```python
from build123d import *

# Parameters (mm, degrees)
F2_R     = 1.55
F2_W     = 2
F2_H     = 2
F3_DEPTH = 1.5
F4_W     = 9
F4_H     = 5
F5_DEPTH = 3
F6_W     = 6
F6_H     = 6.7
F7_DEPTH = 2.5
F6_W_2   = 3.4
F6_H_2   = 3.4
F6_W_3   = 4.4
F6_H_3   = 4.4
F8_DEPTH = 1.5
F6_W_4   = 1.536496
F6_H_4   = 2.176703
F6_H_5   = 2.176704
F6_W_5   = 2.874283
F6_H_6   = 1.806834
F6_W_6   = 2.176703
F6_H_7   = 1.536496
F6_W_7   = 3.137013
F6_H_8   = 2.112682
F9_DEPTH = 2


with BuildPart() as f3:
    # F2 (on Top) → F3 (new body)
    with BuildSketch(Plane.XY):
        Polygon((18, 18), (-18, 18), (-18, 14.369573), (-18, 12.369573), (-18, 10.869573), (-18, 8.869573), (-18, 7.369573), (-18, 5.369573), (-18, 3.005002), (-18, 1.005002), (-18, -0.673528), (-18, -2.673528), (-18, -5.493983), (-18, -7.493983), (-18, -8.993983), (-18, -10.993983), (-18, -12.493983), (-18, -14.493983), (-18, -18), (18, -18), (18, -14.322089), (18, -12.322089), (18, -10.322089), (18, -8.322089), (18, -6.322089), (18, -4.322089), (18, 4.09024), (18, 6.09024), (18, 7.69024), (18, 9.69024), (18, 11.29024), (18, 13.29024), align=None)
        with Locations((-15.25, -15.25)):
            Circle(F2_R, mode=Mode.SUBTRACT)
        with Locations((15.25, -15.25)):
            Circle(F2_R, mode=Mode.SUBTRACT)
        with Locations((-15.25, 15.25)):
            Circle(F2_R, mode=Mode.SUBTRACT)
        with Locations((15.25, 15.25)):
            Circle(F2_R, mode=Mode.SUBTRACT)
        with Locations((-19, 13.369573)):
            Rectangle(F2_W, F2_H)
        with Locations((19, 12.29024)):
            Rectangle(F2_W, F2_H)
        with Locations((-19, 9.869573)):
            Rectangle(F2_W, F2_H)
        with Locations((19, 8.69024)):
            Rectangle(F2_W, F2_H)
        with Locations((-19, 6.369573)):
            Rectangle(F2_W, F2_H)
        with Locations((19, 5.09024)):
            Rectangle(F2_W, F2_H)
        with Locations((-19, 2.005002)):
            Rectangle(F2_W, F2_H)
        with Locations((19, -5.322089)):
            Rectangle(F2_W, F2_H)
        with Locations((-19, -1.673528)):
            Rectangle(F2_W, F2_H)
        with Locations((19, -9.322089)):
            Rectangle(F2_W, F2_H)
        with Locations((-19, -6.493983)):
            Rectangle(F2_W, F2_H)
        with Locations((19, -13.322089)):
            Rectangle(F2_W, F2_H)
        with Locations((-19, -9.993983)):
            Rectangle(F2_W, F2_H)
        with Locations((-19, -13.493983)):
            Rectangle(F2_W, F2_H)
    extrude(amount=F3_DEPTH)

    # F4 (on face) → F5 (join)
    with BuildSketch(Plane.XY.offset(1.5)):
        with Locations((-0.321198, 15.5)):
            Rectangle(F4_W, F4_H)
    extrude(amount=F5_DEPTH)

    # F6 (on face) → F7 (join)
    with BuildSketch(Plane(origin=(0, 0, 0), x_dir=(1, 0, 0), z_dir=(0, 0, -1))):
        with Locations((2.004663, -14.65)):
            Rectangle(F6_W, F6_H)
        with Locations((-7.845552, 14.65)):
            Rectangle(F6_W, F6_H)
        with Locations((7.711476, 14.65)):
            Rectangle(F6_W, F6_H)
    extrude(amount=F7_DEPTH)

    # F6 (on face) → F8 (join)
    with BuildSketch(Plane(origin=(0, 0, 0), x_dir=(1, 0, 0), z_dir=(0, 0, -1))):
        with Locations((-12.063461, -10.042248)):
            Rectangle(F6_W_2, F6_H_2)
        with Locations((-5.725725, -5.885644)):
            Rectangle(F6_W_3, F6_H_3)
        with Locations((6.013899, -6.527154)):
            Rectangle(F6_W_3, F6_H_3)
        with Locations((11.864845, -3.498852)):
            Rectangle(F6_W_2, F6_H_2)
        with Locations((12.121448, 7.278509)):
            Rectangle(F6_W_2, F6_H_2)
        with Locations((6.078051, 4.699263)):
            Rectangle(F6_W_3, F6_H_3)
        with Locations((-5.725725, 5.687943)):
            Rectangle(F6_W_3, F6_H_3)
        with Locations((-11.871008, 4.389598)):
            Rectangle(F6_W_2, F6_H_2)
    extrude(amount=F8_DEPTH)

    # F6 (on face) → F9 (join)
    with BuildSketch(Plane(origin=(0, 0, 0), x_dir=(1, 0, 0), z_dir=(0, 0, -1))):
        with Locations((-9.702151, -4.16677)):
            Rectangle(F6_W_4, F6_H_4)
        with Locations((-9.254006, 7.17795)):
            Rectangle(F6_W_4, F6_H_4)
        with Locations((9.9522, -8.328114)):
            Rectangle(F6_W_4, F6_H_5)
        with Locations((-3.516199, -14.194596)):
            Rectangle(F6_W_5, F6_H_6)
        with Locations((9.888179, 2.235299)):
            Rectangle(F6_W_6, F6_H_7)
        with Locations((-2.17972, 14.495261)):
            Rectangle(F6_W_7, F6_H_8)
        with Locations((2.109666, 14.495261)):
            Rectangle(F6_W_7, F6_H_8)
    extrude(amount=F9_DEPTH)


solid = f3.part
```
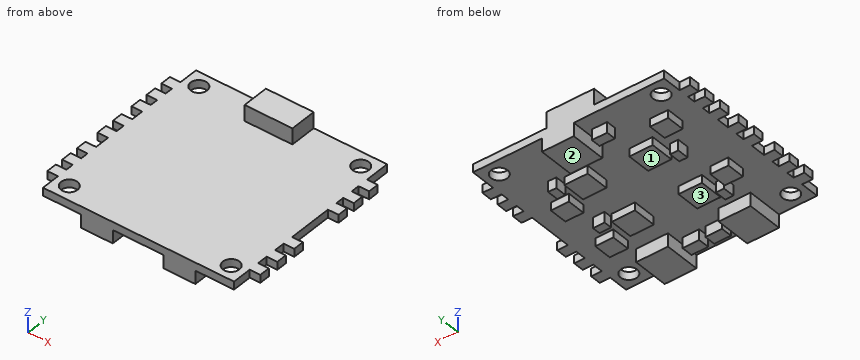
Could you check a few things on this model? Use its own coordinates, in mm. Face numbers are marked on the shaded views. A direction names the side the tool comes from. Coordinates: 2 decimals unless noted, no trailing zeros. Write each loop counter-clockwise with the first axis right and the second up, starting at its lowest first coordinate (ties: lowest second). Pieces come first, ordered by that corner, then holes. Notation, with made-up numbers: (-22.75, 73) -> (24.25, 73) arc R36 cw to (24.25, 112) -> close; hole circle Ø3 at (18.5, 64). An arc over 180 degrees is marked (long way). Return JSON: item names as keys, results as strings.
(1) Imagine slicing it at B-B, the plane y = -13. Please give me the cut outline in (x, z), then the cut area to 3 significant figures.
Numbers:
{"outline": "(-20, 0) -> (-10.85, 0) -> (-10.85, -2.5) -> (-4.85, -2.5) -> (-4.85, 0) -> (4.71, 0) -> (4.71, -2.5) -> (10.71, -2.5) -> (10.71, 0) -> (20, 0) -> (20, 1.5) -> (-20, 1.5) -> close", "area": "90.0 mm2"}
(2) I need wall thicknesses on L1, parallel to Y at x = -15.25, z = 0.6; L2, parallel to X at y = -16, z = 0.5; L3, parallel to Y at x = -11.5, z = -0.5. Which ranges of each line are inside material? Lowest first, please.
Numbers:
{"L1": "y = -18 to -16.8, -13.7 to 13.7, 16.8 to 18", "L2": "x = -18 to -16.61, -13.89 to 13.89, 16.61 to 18", "L3": "y = -6.09 to -2.69, 8.34 to 11.74"}
(3) Which directions (+Z, -Z, +X, -X, +Y, -Y) give clear straight access to the entire face, cutting with the end or side of a thin tool? Please do the marked faces 1, 2 and 3.
Numbers:
{"face 1": "-Z", "face 2": "-Z, +X, -X, +Y, -Y", "face 3": "-Z, +X"}
(4) Imagine slicing it at A-A, the plane x = -15.25. Please give me the cut outline in (y, z).
Numbers:
{"outline": "(-18, 0) -> (-16.8, 0) -> (-16.8, 1.5) -> (-18, 1.5) -> close; (-13.7, 0) -> (13.7, 0) -> (13.7, 1.5) -> (-13.7, 1.5) -> close; (16.8, 0) -> (18, 0) -> (18, 1.5) -> (16.8, 1.5) -> close"}
(5) Imagine slicing it at C-C, the plane x = 3. Please give me the cut outline in (y, z), then the cut area to 3 significant figures.
Numbers:
{"outline": "(-18, 0) -> (-15.55, 0) -> (-15.55, -2) -> (-13.44, -2) -> (-13.44, 0) -> (11.3, 0) -> (11.3, -2.5) -> (18, -2.5) -> (18, 4.5) -> (13, 4.5) -> (13, 1.5) -> (-18, 1.5) -> close", "area": "90.0 mm2"}
(6) I'm going to push flat-ended pins straight in: pin 1 (0.8 mm diameter, centred on x = -19, z = 0.5, fed in from +Y); pin 2 (1.6 mm diameter, centred on y = 8.5, z = -1.5, fed in from -X); pin 3 (1.6 mm diameter, centred on x = -19, z = 1, fed in from -Y). Where does each tip first touch, or does it pass through?
Numbers:
{"pin 1": "stops at y = 14.37", "pin 2": "stops at x = -13.76", "pin 3": "stops at y = -14.49"}
(7) Imagine slicing it at D-D, the plane z = 2. Please give me the cut outline in (x, y).
Numbers:
{"outline": "(-4.82, 13) -> (4.18, 13) -> (4.18, 18) -> (-4.82, 18) -> close"}
